from build123d import *

# Parameters (mm, degrees)
BOSS_EXTRUDE1_DEPTH = 5
SKETCH2_R           = 1.5
BOSS_EXTRUDE2_DEPTH = 6


with BuildPart() as part:
    # Sketch1 → Boss-Extrude1 (new body)
    with BuildSketch(Plane(origin=(0, -9.928470523, 0), x_dir=(1, 0, 0), z_dir=(0, 1, 0))):
        Polygon((52.683579598, -6.935769114), (-2.820579734, -6.935769114), (-7.316420402, -6.935769114), (-7.316420402, -0.935769114), (52.683579598, -0.935769114), align=None)
    extrude(amount=BOSS_EXTRUDE1_DEPTH)

    # Sketch2 → Boss-Extrude2 (add)
    with BuildSketch(Plane.XZ.offset(9.928470523)):
        with Locations((-4.316420402, 3.935769114)):
            Circle(SKETCH2_R)
    extrude(amount=BOSS_EXTRUDE2_DEPTH)


solid = part.part
Read the model definition and answer for the solid it produces. Units are mm, in the model's axes. A direction names the side the tool comes from. Give positions to 0.01 mm unless a question says otherwise; leave off trailing zeros. Write each loop counter-clockwise with the first axis right and the second up, starting at its lowest first coordinate (ties: lowest second). Pieces come first, ordered by that corner, then holes. Notation, with made-up numbers: (22.5, -1) - (59.5, -1) arc R15 cw to (59.5, 22) - close; hole circle Ø11 at (72, 85.5). An arc over 180 degrees is marked (long way). Use CSV: the item, a comma, the result in double quotes. Start each with the question number.
Item 1: The part is cut by section D-D, the plane z = 6.3. Give the vertices of the cut face in (x, y).
Item 2: The part is cut by section B-B, the plane x = 40. Give the vertices of the cut face in (y, z), and give its area (3 significant figures).
Item 3: For faces 1 (the flat face through (22, -7, 0.936)), 2 (the cylindrical face through (-5.507, -12.886, 3.023)), determine the directions among +Z, -Z, +X, -X, +Y, -Y from which every point of the face is accessible in a straight line to the end or side of a thin tool.
Item 4: The part is cut by section C-C, the plane y = -12.75. Give the vertices of the cut face in (x, z).
Item 5: The part is cut by section A-A, the plane z = 3.1. Give the vertices of the cut face in (x, y).
Item 6: Consider line 1 (Y direction, x = 10.5, z = 3.4); line 2 (X direction, y = -10.75, z = 4.1); line 3 (X direction, y = -10.25, z = 3.6). Determine where each line is inside the solid, lowest interval first.
Taken from the geometry:
1,outline,"(-7.32, -9.93) - (52.68, -9.93) - (52.68, -4.93) - (-7.32, -4.93) - close"
2,outline,"(-9.93, 0.94) - (-4.93, 0.94) - (-4.93, 6.94) - (-9.93, 6.94) - close"
2,area,"30.0 mm2"
3,face 1,"-Z, +X, -X, +Y, -Y"
3,face 2,"-Y"
4,outline,"circle Ø3 at (-4.32, 3.94)"
5,outline,"(-7.32, -9.93) - (-5.56, -9.93) - (-5.56, -15.93) - (-3.07, -15.93) - (-3.07, -9.93) - (52.68, -9.93) - (52.68, -4.93) - (-7.32, -4.93) - close"
6,line 1,"-9.93 to -4.93"
6,line 2,"-5.81 to -2.83"
6,line 3,"-5.78 to -2.85"
